Verification items for the finished model (mm, model axes). Give positions to 0.01 mm unless a question says otherwise; leave off trailing zeros. Write each loop counter-clockwise with the first axis right and the second up, starting at its lowest first coordinate (ties: lowest second). Pieces come first, ordered by that corner, then holes. Notation, with made-up numbers: M 55.5,44 L 93.5,44 A29 ccw 93.5,68 Z; hole C 70,36.25 d5. An arc over 180 degrees is marked long. Answer as a JSON object with one key per item and string values.
```python
from build123d import *

# Parameters (mm, degrees)
SKETCH1_W           = 80
SKETCH1_H           = 16.5
BOSS_EXTRUDE1_DEPTH = 3
SKETCH3_W           = 8.2
SKETCH3_H           = 3.2
SKETCH3_W_2         = 16.2
CUT_EXTRUDE1_DEPTH  = 4
FILLET1_R           = 3


with BuildPart() as part:
    # Sketch1 → Boss-Extrude1 (new body)
    with BuildSketch(Plane(origin=(0, 0, 0), x_dir=(1, 0, 0), z_dir=(0, 1, 0))):
        with Locations((40, -8.25)):
            Rectangle(SKETCH1_W, SKETCH1_H)
    extrude(amount=-BOSS_EXTRUDE1_DEPTH)

    # Sketch3 → Cut-Extrude1 (cut, through all)
    with BuildSketch(Plane(origin=(0, 0, 0), x_dir=(1, 0, 0), z_dir=(0, 1, 0))):
        with Locations((8, -9.7)):
            Rectangle(SKETCH3_W, SKETCH3_H)
        with Locations((32, -1.5)):
            Rectangle(SKETCH3_W, SKETCH3_H)
        with Locations((40, -9.7)):
            Rectangle(SKETCH3_W, SKETCH3_H)
        with Locations((24, -9.7)):
            Rectangle(SKETCH3_W, SKETCH3_H)
        with Locations((12, -1.5)):
            Rectangle(SKETCH3_W_2, SKETCH3_H)
        with Locations((48, -1.5)):
            Rectangle(SKETCH3_W, SKETCH3_H)
        with Locations((56, -9.7)):
            Rectangle(SKETCH3_W, SKETCH3_H)
        with Locations((72, -9.7)):
            Rectangle(SKETCH3_W, SKETCH3_H)
        with Locations((68, -1.5)):
            Rectangle(SKETCH3_W_2, SKETCH3_H)
    extrude(amount=-CUT_EXTRUDE1_DEPTH, mode=Mode.SUBTRACT)

    # Fillet1
    fillet1_edges = [part.edges().sort_by_distance(p)[0] for p in [
        (80, -1.5, 16.5),
        (0, -1.5, 16.5),
    ]]
    fillet(fillet1_edges, radius=FILLET1_R)


solid = part.part
```
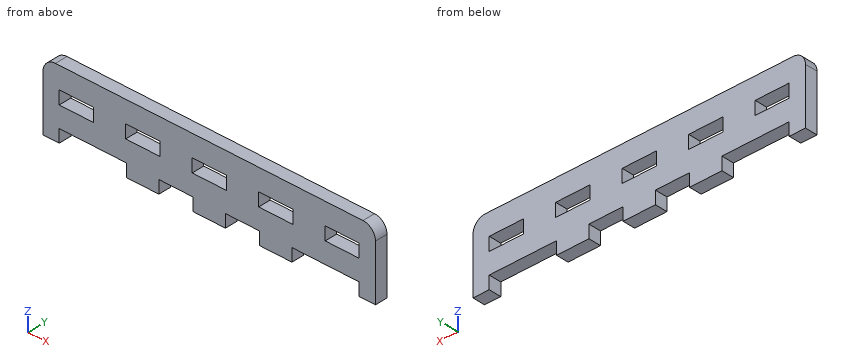
1) Section check A-A on z = 10.5. Record the boundary of the cut face in (x, y), and give its area (3 significant figures).
Completed:
{"outline": "M 0,-3 L 3.9,-3 L 3.9,0 L 0,0 Z; M 12.1,-3 L 19.9,-3 L 19.9,0 L 12.1,0 Z; M 28.1,-3 L 35.9,-3 L 35.9,0 L 28.1,0 Z; M 44.1,-3 L 51.9,-3 L 51.9,0 L 44.1,0 Z; M 60.1,-3 L 67.9,-3 L 67.9,0 L 60.1,0 Z; M 76.1,-3 L 80,-3 L 80,0 L 76.1,0 Z", "area": "117 mm2"}
2) Section check B-B on x = 24. Record the boundary of the cut face in (y, z), and give its area (3 significant figures).
Completed:
{"outline": "M -3,0 L 0,0 L 0,8.1 L -3,8.1 Z; M -3,11.3 L 0,11.3 L 0,16.5 L -3,16.5 Z", "area": "39.9 mm2"}
3) Thickness scan on L1, parallel to X at y = -1.55, z = 2.25; L2, parallel to X at y = -0.5, z = 10.5; L3, parallel to Z at x = 68, y = -1.45. Record the ranges inside material, lowest first.
Completed:
{"L1": "x = 0 to 3.9, 20.1 to 27.9, 36.1 to 43.9, 52.1 to 59.9, 76.1 to 80", "L2": "x = 0 to 3.9, 12.1 to 19.9, 28.1 to 35.9, 44.1 to 51.9, 60.1 to 67.9, 76.1 to 80", "L3": "z = 3.1 to 8.1, 11.3 to 16.5"}
4) Go/stop test with a flat-tipped pin: pin 1 (0.9 mm diameter, centred on x = 8, y = -2, fed in from -Z). Record where the tip stops, or that it passes through.
Completed:
{"pin 1": "stops at z = 3.1"}
5) Section check D-D on x = 74. Record the boundary of the cut face in (y, z).
Completed:
{"outline": "M -3,3.1 L 0,3.1 L 0,8.1 L -3,8.1 Z; M -3,11.3 L 0,11.3 L 0,16.5 L -3,16.5 Z"}
6) Section check C-C on y = -2.55. Count the separate pieces of the cut face and the enclosed holes in it, and give its area (3 significant figures).
Completed:
{"separate pieces": "1", "enclosed holes": "5", "area": "1,030 mm2"}
